Could you check a few things on this drawing? It's one solid part, dimensions in mm from its lowest x, y, z. A direction names the side the tool comes from. Give positions to 0.01 mm unless a question says otherwise; leave off trailing zeros. Loops run counter-clockwise (first coordinate to the right, second up) from the corner with the lowest first, then second, coordinate; pieces in that order, holes last. Notation, with made-up numbers: M 1,1 L 21,1 A24 ccw 21,22 Z; hole C 82,4 d1. An arc over 180 degrees is marked long. Answer in a Markdown table with one row per item. Add a question column.
1. If we section it at B-B on z = 150: List the corners of the cut face in (x, y) for me, then the cut area to 3 significant figures.
2. I need wall thicknesses on line 1 along Z through (x, y) = (19.5, 7); line 2 along Y through (x, z) = (14.75, 150); line 3 along Z through (x, y) = (22, 22). Which ranges of each line are inside material? Lowest first, please. Write a range as from..to.
3. If we section it at A-A on y = 7: List the corners of the cut face in (x, z) for me.
4. I'm going to push flat-ended pins straight in: pin 1 Ø9 at (x, z) = (11, 157) entering from +Y; pin 2 Ø10 at (x, y) = (5, 48) entering from +Z. Where does each tip first touch, or does it pass through?
5. If we section it at C-C on x = 11: List the corners of the cut face in (y, z) for me.
6. If we section it at D-D on z = 18: List the corners of the cut face in (x, y) for me, then the cut area to 3 significant figures.
7. Which directions (+Z, -Z, +X, -X, +Y, -Y) give clear straight access to the entire face, cutting with the end or side of a thin tool? Please do the marked faces 1, 2 and 3.
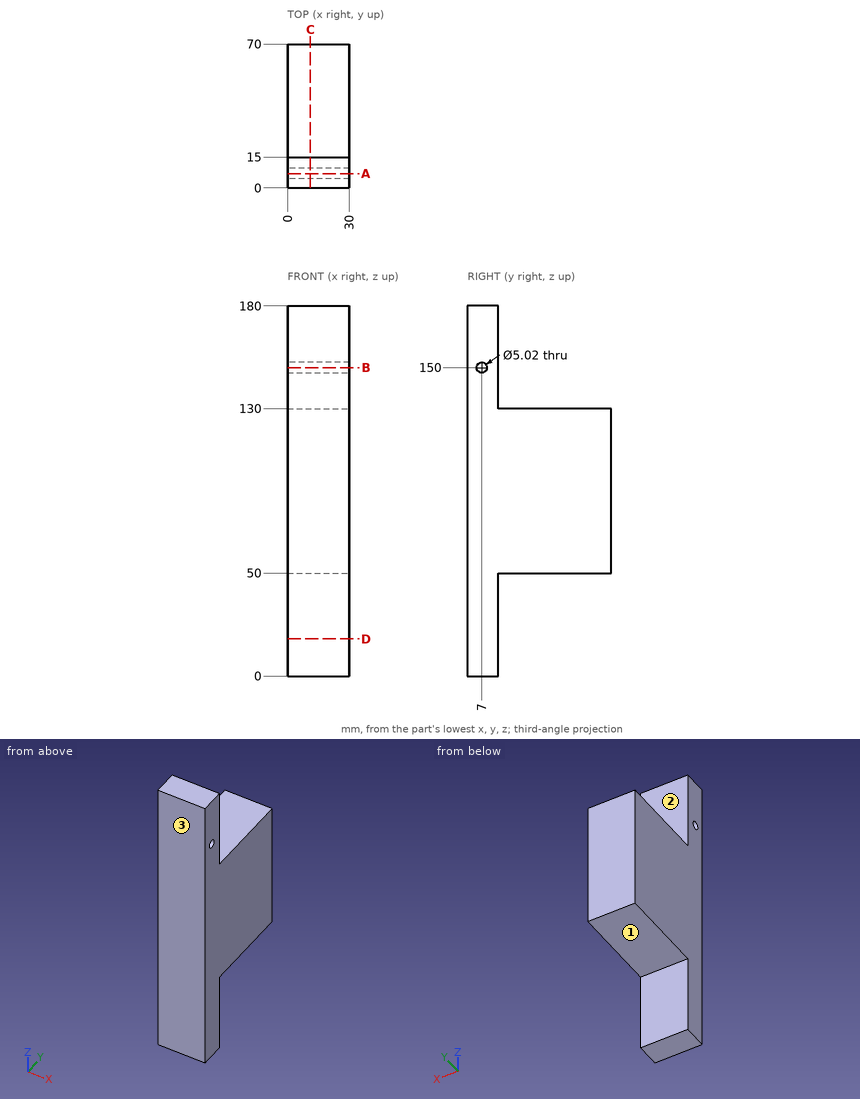
Results:
| question | item | result |
|---|---|---|
| 1 | outline | M 0,0 L 30,0 L 30,4.49 L 0,4.49 Z; M 0,9.51 L 30,9.51 L 30,15 L 0,15 Z |
| 1 | area | 299 mm2 |
| 2 | line 1 | 0..147.49, 152.51..180 |
| 2 | line 2 | 0..4.49, 9.51..15 |
| 2 | line 3 | 50..130 |
| 3 | outline | M 0,0 L 30,0 L 30,147.49 L 0,147.49 Z; M 0,152.51 L 30,152.51 L 30,180 L 0,180 Z |
| 4 | pin 1 | y = 15 |
| 4 | pin 2 | z = 130 |
| 5 | outline | M 0,0 L 15,0 L 15,50 L 70,50 L 70,130 L 15,130 L 15,180 L 0,180 Z; hole C 7,150 d5.02 |
| 6 | outline | M 0,0 L 30,0 L 30,15 L 0,15 Z |
| 6 | area | 450 mm2 |
| 7 | face 1 | -Z, +X, -X, +Y |
| 7 | face 2 | +Z, +X, -X, +Y |
| 7 | face 3 | +Z, -Z, +X, -X, -Y |
